Part model, mm, in its own coordinate system. Face numbers are marked on the shaded views. A direction names the side the tool comes from. Give positions to 0.01 mm unless a question says otherwise; leave off trailing zeros. Order: outer loops, then holes, each group sorted by start corner. A loop starts at its lowest first (then second) coordinate and runs counter-clockwise, first axis right, second up. Notation, with made-up numbers: (-33.5, -30) - (19.5, -30) arc R23 ccw to (19.5, -4) - close; hole circle Ø1 at (-20, 48). An arc over 180 degrees is marked (long way). Use one line per item in the form item = value. Start each with the question number.
1. Band-saw the part on C-C, the plane x = -20.9. List the corners of the cut face in (y, z), plus the area to 3 significant figures.
2. Band-saw the part on A-A, the plane y = 4.45. List the corners of the cut face in (x, z).
3. Pull direction Z, two halves, no side cores. Call the marked faces 6, 7, 8 and 9: +Z half, -Z half, draft (parallel to the pull), parting line (faces both ways), or undercut.
4. Band-saw the part on D-D, the plane z = 10.5. List the corners of the cut face in (x, y).
5. Band-saw the part on B-B, the plane z = 14.75. List the corners of the cut face in (x, y).
6. Tool access for the marked faces 1, 2, 3, 4 and 5: list every direction of +Z, -Z, +X, -X, +Y, -Y with a clear straight run to the whole face (end or side of a thin tool).
7. Pin check, flat tips, straight feed: P1, Ø1, axis at x = -22.5, z = 11, coming from the +Y side; P2, Ø0.6, axis at y = 4, z = 12, coming from the -X side; P3, Ø2, axis at x = -22, y = 1, coming from the +Z side; P4, Ø0.6, axis at y = 1.5, z = 12.5, coming from the +X side. Stop position of each tip, or through.
8. Drill centre lines: line 1 (Y direction, x = -22.9, z = 16.75); line 2 (X direction, y = 4.1, z = 12.5); line 3 (Y direction, x = -22.5, z = 7.5). Where is each one in solid material? Low to high.
from build123d import *

# Parameters (mm, degrees)
BOSS_EXTRUDE1_DEPTH      = 0.508
BOSS_EXTRUDE1_DEPTH_BACK = 0.508
SKETCH1_W                = 3.81
SKETCH1_H                = 16.51
BOSS_EXTRUDE2_DEPTH      = 2.032
BOSS_EXTRUDE2_DEPTH_BACK = 2.54
SKETCH1_3_W              = 2.286
SKETCH1_3_H              = 4.826
FILLET1_R                = 0.254


with BuildPart() as part:
    # Sketch1 → Boss-Extrude1 (new, two sides: drawn at the far end of the back side and taken through both)
    with BuildSketch(Plane(origin=(0, 3.048, 0), x_dir=(1, 0, 0), z_dir=(0, 1, 0)).offset(-BOSS_EXTRUDE1_DEPTH_BACK)):
        with Locations((-21.437752693, -9.378592753)):
            Rectangle(SKETCH1_W, SKETCH1_H)
    extrude(amount=BOSS_EXTRUDE1_DEPTH + BOSS_EXTRUDE1_DEPTH_BACK)

    # Sketch1<3> → Boss-Extrude2 (add, two sides: drawn at the far end of the back side and taken through both)
    with BuildSketch(Plane(origin=(0, 3.048, 0), x_dir=(1, 0, 0), z_dir=(0, 1, 0)).offset(-BOSS_EXTRUDE2_DEPTH_BACK)):
        with Locations((-21.437752693, -5.632092753)):
            Rectangle(SKETCH1_3_W, SKETCH1_3_H)
        with Locations((-21.437752693, -13.125092753)):
            Rectangle(SKETCH1_3_W, SKETCH1_3_H)
    extrude(amount=BOSS_EXTRUDE2_DEPTH + BOSS_EXTRUDE2_DEPTH_BACK)

    # Fillet1
    fillet1_edges = [part.edges().sort_by_distance(p)[0] for p in [
        (-21.437752693, 5.08, 10.712092753),
        (-20.294752693, 5.08, 13.125092753),
        (-22.580752693, 5.08, 13.125092753),
        (-21.437752693, 5.08, 15.538092753),
        (-21.437752693, 5.08, 3.219092753),
        (-20.294752693, 5.08, 5.632092753),
        (-22.580752693, 5.08, 5.632092753),
        (-21.437752693, 5.08, 8.045092753),
    ]]
    fillet(fillet1_edges, radius=FILLET1_R)


solid = part.part
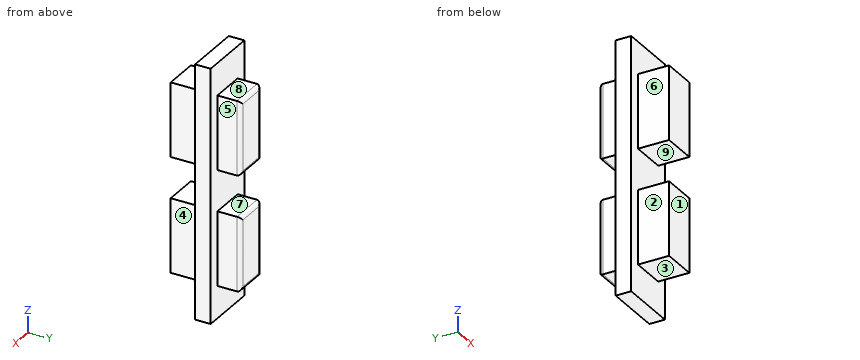
From the geometry:
q1.outline = (0.51, 3.22) - (2.54, 3.22) - (2.54, 1.12) - (3.56, 1.12) - (3.56, 3.22) - (4.83, 3.22) arc R0.25 ccw to (5.08, 3.47) - (5.08, 7.79) arc R0.25 ccw to (4.83, 8.05) - (3.56, 8.05) - (3.56, 10.71) - (4.83, 10.71) arc R0.25 ccw to (5.08, 10.97) - (5.08, 15.28) arc R0.25 ccw to (4.83, 15.54) - (3.56, 15.54) - (3.56, 17.63) - (2.54, 17.63) - (2.54, 15.54) - (0.51, 15.54) - (0.51, 10.71) - (2.54, 10.71) - (2.54, 8.05) - (0.51, 8.05) - close
q1.area = 51.0 mm²
q2.outline = (-22.58, 3.22) - (-20.29, 3.22) - (-20.29, 8.05) - (-22.58, 8.05) - close; (-22.58, 10.71) - (-20.29, 10.71) - (-20.29, 15.54) - (-22.58, 15.54) - close
q3.face_6 = draft
q3.face_7 = undercut
q3.face_8 = +Z half
q3.face_9 = undercut
q4.outline = (-23.34, 2.54) - (-19.53, 2.54) - (-19.53, 3.56) - (-23.34, 3.56) - close
q5.outline = (-23.34, 2.54) - (-22.58, 2.54) - (-22.58, 0.51) - (-20.29, 0.51) - (-20.29, 2.54) - (-19.53, 2.54) - (-19.53, 3.56) - (-20.29, 3.56) - (-20.29, 4.83) arc R0.25 ccw to (-20.55, 5.08) - (-22.33, 5.08) arc R0.25 ccw to (-22.58, 4.83) - (-22.58, 3.56) - (-23.34, 3.56) - close
q6.face_1 = +Z, -Z, +X, -X, -Y
q6.face_2 = +Z, -Z, -X, -Y
q6.face_3 = -Z, +X, -X, -Y
q6.face_4 = +Z, -Z, +X, -Y
q6.face_5 = +Z, -Z, +X, +Y
q7.P1 = 5.08
q7.P2 = -22.58
q7.P3 = 15.54
q7.P4 = -20.29
q8.line_1 = 2.54 to 3.56
q8.line_2 = -22.58 to -20.29
q8.line_3 = 0.51 to 5.01
